The listing builds one solid part. Answer for the finished solid, in the listing's coordinates (mm). A direction names the side the tool comes from. Round coordinates to 2 decimals unless told otherwise and drop trailing zeros. Order: outer loops, then holes, each group sorted by start corner. A loop starts at its lowest first (then second) coordinate and runs counter-clockwise, first axis right, second up. Notation, with made-up numbers: (-2, -6) - (38, -6) arc R36 cw to (38, 31) - close; hole circle Ø6 at (76, -36). An arc over 180 degrees is marked (long way). One line per item, written item: value. Start each with the question number.
1. For a pull along X with two mould halves and no side action, classify faces 4 (the flat face through (-46, 0, -60)), 5 (the cylindrical face through (-100.49, 6.2, -60.72)), 6 (the flat face through (0, 0, 87)), 7 (the cylindrical face through (-13.004, -0.035, 148.736)) as released by +X, released by -X, zero draft, split by the parting line, or undercut.
2. Flat-ended cylindrical pins translate along their axes: P1, Ø3, axis at x = -67.5, y = 8, coming from the -Z side; P2, Ø12, axis at x = -110.5, y = -0.5, coming from the +Z side; P3, Ø2, axis at x = -111.5, z = -45.5, coming from the +Y side. Find the tip coordinate at first contact, or state that the pin passes through.
3. Section C-C, the plane x = -20 is taken. Count the separate pieces of the cut face and the enclosed holes in it, then the cut area to 3 significant figures.
4. A tool of negligible diameter and unlimited length cuts with its end or side. For faces 1 (the flat face through (-46, -6, -95)), 2 (the flat face through (-113, -2.5, -1)), 3 (the flat face through (-46, 6, -65)), from which of +Z, -Z, +X, -X, +Y, -Y can it reach the whole face along a straight path? Write none if from no direction.
5. Section A-A, the plane y = 5.5 is taken. Give the vertices of the cut face in (x, z).
6. Straight lines are drawn through the part: line 1 (Z direction, x = -20, y = -0.9); line 2 (Z direction, x = -67, y = -6.25); line 3 (X direction, y = 4.5, z = -30.5). For each, find the intervals that lie inside material, in ascending order.
7. Section B-B, the plane z = 8.5 is taken. Give the vertices of the cut face in (x, y).
8. Section D-D, the plane x = -124.5 is taken. Give the vertices of the cut face in (y, z), then the cut area to 3 significant figures.
from build123d import *

# Parameters (mm, degrees)
F3_R     = 5
F4_DEPTH = 2.5


with BuildPart() as f2:
    # F2: sweep along a path in F0
    with BuildLine(Plane.XZ) as f2_path:
        Line((0, 60), (-90, 60))
        ThreePointArc((-90, 60), (-97.071068, 57.071068), (-100, 50))
        Line((-100, 50), (-100, 0))
    # F1 (on Right) → F2 (sweep)
    with BuildSketch(Plane.YZ):
        Polygon((-10, 60), (0, 60), (10, 60), (10, 65), (2.5, 65), (2.5, 95), (10, 95), (10, 100), (0, 100), (-10, 100), (-10, 95), (-2.5, 95), (-2.5, 65), (-10, 65), align=None)
    sweep(path=f2_path.line)

    # F3 (on Front) → F4 (join, symmetric)
    with BuildSketch(Plane.XZ):
        with BuildLine():
            Line((-70, 100), (0, 100))
            Line((0, 100), (0, 130))
            ThreePointArc((0, 130), (-13.327703, 148.854189), (-35.548045, 142.580075))
            Line((-35.548045, 142.580075), (-70, 100))
        make_face()
        with Locations((-20, 130)):
            Circle(F3_R, mode=Mode.SUBTRACT)
    extrude(amount=F4_DEPTH, both=True)

    # F5: F2 across plane


with BuildPart() as f2_1:
    add(f2.part)
    add(f2.part.mirror(Plane.XY))


solid = f2_1.part
Answer list:
1. face 4: zero draft
1. face 5: undercut
1. face 6: released by +X
1. face 7: split by the parting line
2. P1: stops at z = -100
2. P2: stops at z = 97.85
2. P3: stops at y = 2.5
3. separate pieces: 4
3. enclosed holes: 0
3. area: 1,100 mm²
4. face 1: +X, -Y
4. face 2: -Y
4. face 3: +X, +Y
5. outline: (-140, -50) arc R50 ccw to (-90, -100) - (0, -100) - (0, -95) - (-90, -95) arc R45 cw to (-135, -50) - (-135, 50) arc R45 cw to (-90, 95) - (0, 95) - (0, 100) - (-90, 100) arc R50 ccw to (-140, 50) - close; (-105, -50) arc R15 ccw to (-90, -65) - (0, -65) - (0, -60) - (-90, -60) arc R10 cw to (-100, -50) - (-100, 50) arc R10 cw to (-90, 60) - (0, 60) - (0, 65) - (-90, 65) arc R15 ccw to (-105, 50) - close
6. line 1: z = -150 to -135, -125 to -60, 60 to 125, 135 to 150
6. line 2: z = -100 to -95, -65 to -60, 60 to 65, 95 to 100
6. line 3: x = -140 to -135, -105 to -100
7. outline: (-140, -10) - (-135, -10) - (-135, -2.5) - (-105, -2.5) - (-105, -10) - (-100, -10) - (-100, 10) - (-105, 10) - (-105, 2.5) - (-135, 2.5) - (-135, 10) - (-140, 10) - close
8. outline: (-10, -86.19) - (10, -86.19) - (10, -78.89) - (2.5, -78.89) - (2.5, 78.89) - (10, 78.89) - (10, 86.19) - (-10, 86.19) - (-10, 78.89) - (-2.5, 78.89) - (-2.5, -78.89) - (-10, -78.89) - close
8. area: 1,080 mm²
